Model file for the job. Use its own axes, mm. A direction names the side the tool comes from. Coordinates: 2 decimals unless noted, no trailing zeros. Write each loop counter-clockwise with the first axis right and the second up, starting at its lowest first coordinate (ties: lowest second). Pieces come first, ordered by that corner, then holes. Notation, with made-up numbers: M 23,-18.5 L 38,-18.5 A31 cw 38,10.5 Z; hole C -25,-6 d11. An arc over 180 degrees is marked long. Put each result on its own line as item: value. Start each with the question number.
Q1. Cut at D-D (x = -17.5). Write the cut outline in (y, z), then the cut area to 3 significant figures.
Q2. Cut at C-C (y = -5.75). Write the cut outline in (x, z).
Q3. Cut at A-A (x = -2.55). Write the cut outline in (y, z), then the cut area to 3 significant figures.
Q4. Pull direction Z, two halves, no side cores. Call faces 6 (the cylindrical face through (23.1, -5.7, -1)), 7 (the flat face through (1, 13, -20)), 8 (the cylindrical face through (15.386, -1.014, -15.239)), 9 (the flat face through (34, 19, -1.3)): pulls with the +Z half, pulls with the -Z half, needs draft (parallel to the pull), parting line crosses it, or undercut.
Q5. Drill centre lines: line 1 along X through (y, z) = (-1.1, -16); line 2 along Y through (x, z) = (24.5, -5); line 3 along Z through (x, y) = (-2.55, -0.8). Where is each one in solid material? Low to high.
Q6. Cut at B-B (z = -10). Write the cut outline in (x, y).
Q7. Drop flat-ended pins along their axis: pin 1 (8 mm diameter, centred on x = 27.5, z = -11.5, fed in from -Y); pin 2 (12 mm diameter, centred on x = 12.5, y = 16, fed in from +Z); pin 3 (6 mm diameter, centred on x = 27.5, y = -0.5, fed in from +Z); pin 4 (12 mm diameter, centred on x = 4, z = -5, fed in from -Y). Give the stop position or say it passes through.
Q8. Which spindle directions (+Z, -Z, +X, -X, +Y, -Y) get a long thin tool onto all of the face, cutting with end or side? Do faces 1 (the flat face through (27.5, 11, -21)), 2 (the cylindrical face through (-3.182, -1.014, -14.476)), 3 (the flat face through (-19, -7.85, -1)), 4 (the flat face through (0, -5, 0)), 5 (the flat face through (0, -2, -12)). Say none if no direction does.
```python
from build123d import *

# Parameters (mm, degrees)
EXTRUDE_THIN2_DEPTH     = 27.5
CUT_EXTRUDE4_DEPTH      = 46.053967639
CUT_EXTRUDE4_DEPTH_BACK = 46.053967639
SKETCH6_R               = 1.65
SKETCH8_W               = 8
SKETCH8_H               = 15
BOSS_EXTRUDE1_DEPTH     = 1.5
CUT_EXTRUDE5_DEPTH      = 1.5
FILLET2_R               = 4
FILLET3_R               = 0.25
CUT_EXTRUDE7_DEPTH      = 10
FILLET5_R               = 1


with BuildPart() as part:
    # Sketch1 → Extrude-Thin2 (new, symmetric)
    with BuildSketch(Plane(origin=(0, 0, 0), x_dir=(0, 0, -1), z_dir=(1, 0, 0))):
        Polygon((-0.2, 26.1), (20, 26.1), (20, 0), (0, 0), (0, -9.5), (2, -9.5), (2, -2), (22, -2), (22, 28.1), (-0.2, 28.1), align=None)
    extrude(amount=EXTRUDE_THIN2_DEPTH, both=True)

    # Sketch6 → Cut-Extrude4 (cut, two sides: drawn at the far end of the back side and taken through both)
    with BuildSketch(Plane(origin=(0, 0, 0), x_dir=(1, 0, 0), z_dir=(0, 1, 0)).offset(-CUT_EXTRUDE4_DEPTH_BACK)):
        with Locations(Location((-2.55, 16, 0), (0, 0, 270))):
            Circle(SKETCH6_R)
        with Locations(Location((16.85, 16, 0), (0, 0, 270))):
            Circle(SKETCH6_R)
    extrude(amount=CUT_EXTRUDE4_DEPTH + CUT_EXTRUDE4_DEPTH_BACK, mode=Mode.SUBTRACT)

    # Sketch8 → Boss-Extrude1 (add)
    with BuildSketch(Plane.XY.offset(0.2)):
        with Locations((31.5, 20.6)):
            Rectangle(SKETCH8_W, SKETCH8_H)
    extrude(amount=-BOSS_EXTRUDE1_DEPTH)

    # Sketch9 → Cut-Extrude5 (cut)
    with BuildSketch(Plane(origin=(0, 0, 0.2), x_dir=(-1, 0, 0), z_dir=(0, 0, -1))):
        with BuildLine():
            Line((-29.4, 18), (-29.4, 23))
            ThreePointArc((-29.4, 23), (-31.5, 25.1), (-33.6, 23))
            Line((-33.6, 23), (-33.6, 18))
            ThreePointArc((-33.6, 18), (-31.5, 15.9), (-29.4, 18))
        make_face()
    extrude(amount=CUT_EXTRUDE5_DEPTH, mode=Mode.SUBTRACT)

    # Fillet2
    fillet2_edges = [part.edges().sort_by_distance(p)[0] for p in [
        (27.5, 27.1, -1.3),
    ]]
    fillet(fillet2_edges, radius=FILLET2_R)

    # Fillet3
    fillet3_edges = [part.edges().sort_by_distance(p)[0] for p in [
        (-27.5, -4.75, 0),
        (-27.5, 0, -10),
        (-27.5, 13.05, -20),
        (-27.5, 26.1, -9.9),
        (-27.5, 27.1, 0.2),
        (-27.5, 28.1, -10.9),
        (0, 28.1, -22),
        (0, -2, -22),
        (0, -2, -2),
        (0, -9.5, -2),
        (0, -9.5, 0),
        (0, 0, 0),
        (4, 28.1, 0.2),
        (27.5, 0, -10),
        (27.5, -4.75, 0),
        (27.5, -9.5, -1),
        (27.5, -5.75, -2),
        (27.5, -2, -12),
        (27.5, 13.05, -22),
        (33.5, 28.1, -1.3),
        (35.5, 20.6, -1.3),
        (35.5, 28.1, -0.55),
        (31.5, 13.1, -1.3),
        (35.5, 13.1, -0.55),
        (31.5, 13.1, 0.2),
        (35.5, 20.6, 0.2),
        (27.5, 28.1, -13.65),
        (28.671572875, 28.1, -2.471572875),
        (-27.5, 13.05, -22),
        (-27.5, -2, -12),
        (-27.5, -5.75, -2),
        (-27.5, -9.5, -1),
    ]]
    fillet(fillet3_edges, radius=FILLET3_R)

    # Sketch11 → Cut-Extrude7 (cut)
    with BuildSketch(Plane(origin=(0, 0, -2), x_dir=(-1, 0, 0), z_dir=(0, 0, -1))):
        with BuildLine():
            Line((-21, -7.85), (-16, -7.85))
            ThreePointArc((-16, -7.85), (-13.9, -5.75), (-16, -3.65))
            Line((-16, -3.65), (-21, -3.65))
            ThreePointArc((-21, -3.65), (-23.1, -5.75), (-21, -7.85))
        make_face()
        with BuildLine():
            Line((16, -3.65), (21, -3.65))
            ThreePointArc((21, -3.65), (23.1, -5.75), (21, -7.85))
            Line((21, -7.85), (16, -7.85))
            ThreePointArc((16, -7.85), (13.9, -5.75), (16, -3.65))
        make_face()
    extrude(amount=-CUT_EXTRUDE7_DEPTH, mode=Mode.SUBTRACT)

    # Fillet5
    fillet5_edges = [part.edges().sort_by_distance(p)[0] for p in [
        (29.5, 26.1, -1.3),
    ]]
    fillet(fillet5_edges, radius=FILLET5_R - 0.0001)  # a hair under: the kernel refuses the full size


solid = part.part
```
Computed values:
1. outline: M -9.5,-1.75 A0.25 ccw -9.25,-2 L -7.85,-2 L -7.85,0 L -9.25,0 A0.25 ccw -9.5,-0.25 Z; M -3.65,-2 L -2.25,-2 A0.25 cw -2,-2.25 L -2,-21.75 A0.25 ccw -1.75,-22 L 27.85,-22 A0.25 ccw 28.1,-21.75 L 28.1,-0.05 A0.25 ccw 27.85,0.2 L 26.1,0.2 L 26.1,-20 L 0,-20 L 0,-0.25 A0.25 ccw -0.25,0 L -3.65,0 Z
1. area: 147 mm2
2. outline: M -27.5,-1.75 A0.25 ccw -27.25,-2 L -23.1,-2 L -23.1,0 L -27.25,0 A0.25 ccw -27.5,-0.25 Z; M -13.9,-2 L 13.9,-2 L 13.9,0 L -13.9,0 Z; M 23.1,-2 L 27.25,-2 A0.25 ccw 27.5,-1.75 L 27.5,-0.25 A0.25 ccw 27.25,0 L 23.1,0 Z
3. outline: M -9.5,-1.75 A0.25 ccw -9.25,-2 L -2.25,-2 A0.25 cw -2,-2.25 L -2,-14.35 L 0,-14.35 L 0,-0.25 A0.25 ccw -0.25,0 L -9.25,0 A0.25 ccw -9.5,-0.25 Z; M -2,-21.75 A0.25 ccw -1.75,-22 L 27.85,-22 A0.25 ccw 28.1,-21.75 L 28.1,-17.65 L 26.1,-17.65 L 26.1,-20 L 0,-20 L 0,-17.65 L -2,-17.65 Z; M 26.1,-14.35 L 28.1,-14.35 L 28.1,-0.05 A0.25 ccw 27.85,0.2 L 26.1,0.2 Z
3. area: 142 mm2
4. face 6: needs draft
4. face 7: pulls with the +Z half
4. face 8: undercut
4. face 9: pulls with the -Z half
5. line 1: -27.5 to -4.2, -0.9 to 15.2, 18.5 to 27.5
5. line 2: -2 to 0, 26.1 to 28.1
5. line 3: -22 to -17.65, -14.35 to 0
6. outline: M -27.5,-1.75 A0.25 ccw -27.25,-2 L 27.25,-2 A0.25 ccw 27.5,-1.75 L 27.5,-0.25 A0.25 ccw 27.25,0 L -27.25,0 A0.25 ccw -27.5,-0.25 Z; M -27.5,26.35 A0.25 ccw -27.25,26.1 L 27.5,26.1 L 27.5,27.85 A0.25 ccw 27.25,28.1 L -27.25,28.1 A0.25 ccw -27.5,27.85 Z
7. pin 1: y = -2
7. pin 2: z = -20
7. pin 3: z = 0
7. pin 4: y = -9.5
8. face 1: -Z, +X, -Y
8. face 2: +Y, -Y
8. face 3: +Z, -Z
8. face 4: +Z, +X, -X, -Y
8. face 5: -Z, +X, -X, -Y
